For this review, take the finished solid that the model builds, in its own axes (mm). A direction names the side the tool comes from. Give positions to 0.01 mm unless a question says otherwise; leave off trailing zeros. Write each loop counter-clockwise with the first axis right and the second up, starting at its lowest first coordinate (ties: lowest second). Pieces come first, ordered by that corner, then holes.
Q1. We need section B-B (y = -15). Write out the cut boundary in (x, z), then the cut area to 3 significant figures.
Q2. Machinability: for faces 1 (the flat face through (3, -17, 6.35)), 2 (the flat face through (3, -19, -23.262)), 3 (the cylindrical face through (3.2, -57.8, 22.3)), which of the approach directions +Z, -Z, +X, -X, +Y, -Y give a long, thin tool a straight path to every point of the face, cutting with its end or side? Answer none if there is none.
Q3. We need section C-C (z = -35.5). Write out the cut boundary in (x, y).
Q4. For line 1 (Z direction, x = 3.75, y = -2); line 2 (Z direction, x = 3, y = -8.5), list the stretches that pass through material, from the lowest coordinate up.
Q5. We need section A-A (x = 5.25). Give the number of separate pieces and of enclosed holes in the cut face, then the cut area to 3 significant figures.
Q6. Mouldability with a two-part tool opening along Y and no side actions: class faces 4 (the cylindrical face through (3.13, -0.88, -19.02)), 5 (the cylindrical face through (3.13, -2.23, 0.5)), 6 (the cylindrical face through (3.22, 4.54, -21.35)), 7 (the flat face through (6.35, -34, -5)) as released by +Y, released by -Y, zero draft, split by the parting line, or undercut.
Q7. Insertion check: P1, Ø12, axis at y = -43.5, z = -39, coming from the -X side. The pin has a flat end and moves straight along its axis. Give the tip position at first contact, or say it passes through.
```python
from build123d import *

# Parameters (mm, degrees)
SKETCH1_R           = 2.286
BOSS_EXTRUDE1_DEPTH = 6.35
FILLET1_R           = 12.7
FILLET2_R           = 6.35
FILLET3_R           = 2.54
CUT_EXTRUDE1_DEPTH  = 85.366399734
FILLET4_R           = 25.4


with BuildPart() as part:
    # Sketch1 → Boss-Extrude1 (new body)
    with BuildSketch(Plane(origin=(0, 0, 0), x_dir=(0, 0, -1), z_dir=(1, 0, 0))):
        Polygon((-6.35, 6.35), (-6.35, -46.99), (-24.13, -46.99), (-24.13, -59.69), (67.711814614, -59.69), (23.261814614, -46.99), (23.261814614, 6.35), align=None)
        Circle(SKETCH1_R, mode=Mode.SUBTRACT)
        with Locations((16.911814614, 0)):
            Circle(SKETCH1_R, mode=Mode.SUBTRACT)
    extrude(amount=BOSS_EXTRUDE1_DEPTH)

    # Fillet1
    fillet1_edges = [part.edges().sort_by_distance(p)[0] for p in [
        (3.175, -46.99, -23.261814614),
        (3.175, -46.99, 6.35),
    ]]
    fillet(fillet1_edges, radius=FILLET1_R)

    # Fillet2
    fillet2_edges = [part.edges().sort_by_distance(p)[0] for p in [
        (3.175, 6.35, 6.35),
        (3.175, 6.35, -23.261814614),
        (3.175, -59.69, 24.13),
        (3.175, -46.99, 24.13),
    ]]
    fillet(fillet2_edges, radius=FILLET2_R)

    # Fillet3
    fillet3_edges = [part.edges().sort_by_distance(p)[0] for p in [
        (3.175, -59.69, -67.711814614),
    ]]
    fillet(fillet3_edges, radius=FILLET3_R)

    # Sketch2 → Cut-Extrude1 (cut, through all)
    with BuildSketch(Plane.XZ.offset(59.69)):
        Polygon((0, -41.956075055), (3.175, -52.116075055), (0, -52.116075055), align=None)
    extrude(amount=-CUT_EXTRUDE1_DEPTH, mode=Mode.SUBTRACT)

    # Fillet4
    fillet4_edges = [part.edges().sort_by_distance(p)[0] for p in [
        (0, -56.010608634, -41.956075055),
    ]]
    fillet(fillet4_edges, radius=FILLET4_R)


solid = part.part
```
Computed:
1. outline: (0, -23.26) - (6.35, -23.26) - (6.35, 6.35) - (0, 6.35) - close
1. area: 188 mm2
2. face 1: +Z, +X, -X, +Y
2. face 2: -Z, +X, -X, +Y
2. face 3: +Z, +X, -X, -Y
3. outline: (0, -59.69) - (6.35, -59.69) - (6.35, -50.49) - (0, -50.49) - close
4. line 1: z = -23.26 to -18.02, -15.8 to -1.11, 1.11 to 6.35
4. line 2: z = -23.26 to 6.35
5. separate pieces: 1
5. enclosed holes: 2
5. area: 2,410 mm2
6. face 4: undercut
6. face 5: undercut
6. face 6: released by +Y
6. face 7: zero draft
7. P1: passes through
